Input: part model. Units: mm. Frame: model coordinates. Round coordinates to 2 decimals unless told otherwise and drop trailing zeros. One line per question, with ' | ' between items. Start each with the question number.
Item 1: Material intervals for line 1 along Y through (x, z) = (34.45, -6.35); line 2 along Y through (x, z) = (20.25, -2.4); line 3 along X through (y, z) = (33, -2.55), sorted ascending.
Item 2: First-contact query: pin 1 (0.8 mm diameter, centred on x = 28.5, y = 27, fed in from -Z); pin 2 (1.5 mm diameter, centred on y = 10, z = -6.35, fed in from +X); pin 3 (2 mm diameter, centred on y = 30, z = -6.35, fed in from +X). Flat tips, straight axial feed; report the tip coordinate or a pass-through.
Item 3: Section A-A, the plane z = -9.75. Give the number of separate pieces and of enclosed holes in the cut face, plus the area to 3 significant figures.
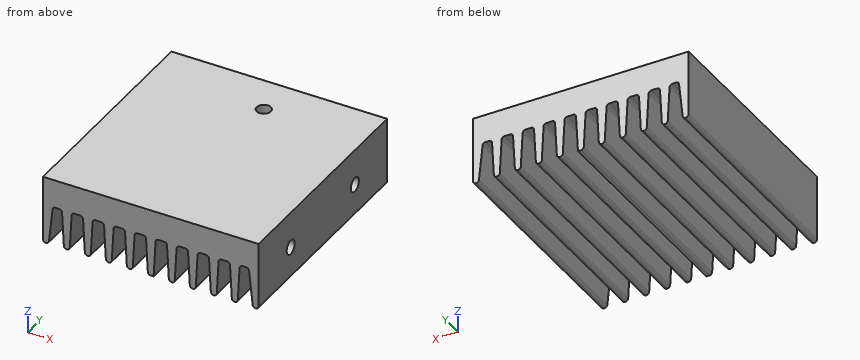
```python
from build123d import *

# Parameters (mm, degrees)
EXTRUDE1_DEPTH            = 40
BOSS_EXTRUDE1_DEPTH       = 40
LPATTERN1_COUNT           = 9
LPATTERN1_PITCH           = 3.7
FILLET1_R                 = 0.5
FILLET2_R                 = 0.5
M3X0_5_TAPPED_HOLE1_D     = 2.5
M3X0_5_TAPPED_HOLE1_DEPTH = 6.5
M3X0_5_TAPPED_HOLE1_TIP   = 0.751075774
M3X0_5_TAPPED_HOLE2_D     = 2.5
M3X0_5_TAPPED_HOLE2_DEPTH = 5
M3X0_5_TAPPED_HOLE2_TIP   = 0.751075774


with BuildPart() as part:
    # Sketch1 → Extrude1 (new body)
    with BuildSketch(Plane(origin=(0, 0, 0), x_dir=(1, 0, 0), z_dir=(0, 1, 0))):
        Polygon((0, 12), (0, 0), (38, 0), (38, 12), (37, 12), (36.264270353, 5), (1.735729647, 5), (1, 12), align=None)
    extrude(amount=EXTRUDE1_DEPTH)

    # Sketch3 → Boss-Extrude1 (add)
    with BuildSketch(Plane(origin=(0, 40, 0), x_dir=(1, 0, 0), z_dir=(0, 1, 0))):
        Polygon((3.333145545, 5), (3.7, 12), (4.7, 12), (5.066854455, 5), align=None)
    boss_extrude1 = extrude(amount=-BOSS_EXTRUDE1_DEPTH)

    # LPattern1: Boss-Extrude1 ×9
    with Locations(*[(i * LPATTERN1_PITCH, 0, 0) for i in range(1, LPATTERN1_COUNT)]):
        add(boss_extrude1)

    # Fillet1
    fillet1_edges = [part.edges().sort_by_distance(p)[0] for p in [
        (34.666854455, 20, -5),
        (32.933145545, 20, -5),
        (1.735729647, 20, -5),
        (36.264270353, 20, -5),
        (5.066854455, 20, -5),
        (3.333145545, 20, -5),
        (8.766854455, 20, -5),
        (7.033145545, 20, -5),
        (12.466854455, 20, -5),
        (10.733145545, 20, -5),
        (16.166854455, 20, -5),
        (14.433145545, 20, -5),
        (19.866854455, 20, -5),
        (18.133145545, 20, -5),
        (23.566854455, 20, -5),
        (21.833145545, 20, -5),
        (27.266854455, 20, -5),
        (25.533145545, 20, -5),
        (30.966854455, 20, -5),
        (29.233145545, 20, -5),
    ]]
    fillet(fillet1_edges, radius=FILLET1_R)

    # Fillet2
    fillet2_edges = [part.edges().sort_by_distance(p)[0] for p in [
        (33.3, 20, -12),
        (34.3, 20, -12),
        (1, 20, -12),
        (37, 20, -12),
        (38, 20, -12),
        (0, 20, -12),
        (3.7, 20, -12),
        (4.7, 20, -12),
        (7.4, 20, -12),
        (8.4, 20, -12),
        (11.1, 20, -12),
        (12.1, 20, -12),
        (14.8, 20, -12),
        (15.8, 20, -12),
        (18.5, 20, -12),
        (22.2, 20, -12),
        (23.2, 20, -12),
        (25.9, 20, -12),
        (26.9, 20, -12),
        (29.6, 20, -12),
        (30.6, 20, -12),
    ]]
    fillet(fillet2_edges, radius=FILLET2_R)

    # M3x0.5 Tapped Hole1
    with Locations(Plane(origin=(38, 0, 0), x_dir=(0, 0, -1), z_dir=(1, 0, 0))):
        with Locations((6.35, 30), (6.35, 10)):
            Hole(M3X0_5_TAPPED_HOLE1_D / 2, depth=M3X0_5_TAPPED_HOLE1_DEPTH)
            with Locations((0, 0, -(M3X0_5_TAPPED_HOLE1_DEPTH + M3X0_5_TAPPED_HOLE1_TIP / 2))):  # 118° drill point
                Cone(0, M3X0_5_TAPPED_HOLE1_D / 2, M3X0_5_TAPPED_HOLE1_TIP, mode=Mode.SUBTRACT)

    # M3x0.5 Tapped Hole2
    with Locations(Plane.XY):
        with Locations((20.25, 33)):
            Hole(M3X0_5_TAPPED_HOLE2_D / 2, depth=M3X0_5_TAPPED_HOLE2_DEPTH)
            with Locations((0, 0, -(M3X0_5_TAPPED_HOLE2_DEPTH + M3X0_5_TAPPED_HOLE2_TIP / 2))):  # 118° drill point
                Cone(0, M3X0_5_TAPPED_HOLE2_D / 2, M3X0_5_TAPPED_HOLE2_TIP, mode=Mode.SUBTRACT)


solid = part.part
```
Return value:
1) line 1: 0 to 8.75, 11.25 to 28.75, 31.25 to 40 | line 2: 0 to 31.75, 34.25 to 40 | line 3: 0 to 19, 21.5 to 38
2) pin 1: z = -5.02 | pin 2: x = 30.94 | pin 3: x = 30.96
3) separate pieces: 11 | enclosed holes: 0 | area: 544 mm2
